Autodesk Inventor part; units mm, degrees
ref_plane "YZ Plane" through (0, 0, 0) normal (1, 0, 0) x (0, 1, 0)
ref_plane "XZ Plane" through (0, 0, 0) normal (0, 1, 0) x (-1, 0, 0)
ref_plane "XY Plane" through (0, 0, 0) normal (0, 0, 1) x (1, 0, 0)
sketch "Skizze1" plane through (0, 0, 0) normal (0, 0, 1) x (1, 0, 0)
  circle A0 centre (0.0001, -0.0022) radius 3.9802
  circle A1 centre (-8.37, 7.9978) radius 1.4
  circle A2 centre (8.3745, -8.0022) radius 1.4
  line L0 (-9.5383, 7.2264) -> (-3.2198, -2.3418)
  line L1 (-7.6522, 9.1998) -> (1.8915, 3.4999)
  line L2 (9.5428, -7.2307) -> (3.3215, 2.191)
  line L3 (-1.8517, -3.5253) -> (7.6567, -9.2041)
  point P0 (0, 0)
extrude "Extrusion1" add sketch "Skizze1" along normal blind 8
sketch "Skizze2" plane through (0, 0, 8) normal (0, 0, 1) x (1, 0, 0)
  arc A0 (-7.6522, 9.1998) -> (-9.5383, 7.2264) centre (-8.37, 7.9978) ccw
  line L0 (-9.5383, 7.2264) -> (-3.2198, -2.3418)
  arc A1 (-3.2198, -2.3418) -> (-1.8517, -3.5253) centre (0.0001, -0.0022) ccw
  line L1 (-1.8517, -3.5253) -> (7.6567, -9.2041)
  arc A2 (7.6567, -9.2041) -> (9.5428, -7.2307) centre (8.3745, -8.0022) ccw
  line L2 (9.5428, -7.2307) -> (3.3215, 2.191)
  arc A3 (3.3215, 2.191) -> (1.8915, 3.4999) centre (0.0001, -0.0022) ccw
  line L3 (1.8915, 3.4999) -> (-7.6522, 9.1998)
  arc A4 (-6.6267, 10.9169) -> (-11.2072, 6.1243) centre (-8.37, 7.9978) ccw
  line L4 (-11.2072, 6.1243) -> (-4.8666, -3.4774)
  arc A5 (-4.8666, -3.4774) -> (-2.8352, -5.2674) centre (0.0001, -0.0022) ccw
  line L5 (-2.8352, -5.2674) -> (6.6312, -10.9212)
  arc A6 (6.6312, -10.9212) -> (11.2118, -6.1287) centre (8.3745, -8.0022) ccw
  line L6 (11.2118, -6.1287) -> (4.9905, 3.2931)
  arc A7 (4.9905, 3.2931) -> (2.8837, 5.2369) centre (0.0001, -0.0022) ccw
  line L7 (2.8837, 5.2369) -> (-6.6267, 10.9169)
  point P0 (0, 0)
  dimension "d2" = 2
extrude "Extrusion2" add sketch "Skizze2" against normal up to surface (8 mm away)
sketch "Skizze3" plane through (0, 0, 8) normal (0, 0, 1) x (1, 0, 0)
  circle A0 centre (0.0001, -0.0022) radius 3.9802
  circle A1 centre (-8.37, 7.9978) radius 1.4
  circle A2 centre (8.3745, -8.0022) radius 1.4
  circle A3 centre (0.0001, -0.0022) radius 3.35
  point P0 (0, 0)
  dimension "d5" = 6.7
extrude "Extrusion3" cut sketch "Skizze3" against normal through all contours A1 | A2 | A3
sketch "Skizze4" plane through (0, 0, 8) normal (0, 0, 1) x (1, 0, 0)
  circle A0 centre (-8.37, 7.9978) radius 1.4
  circle A1 centre (8.3745, -8.0022) radius 1.4
  point P0 (0, 0)
hole "Bohrung1" at (-8.37, 7.9978, 8) at (8.3745, -8.0022, 8) direction (0, 0, -1) diameter 2.8 end through all counterbore diameter 8 counterbore depth 6
properties part number "IM_Lensholder"
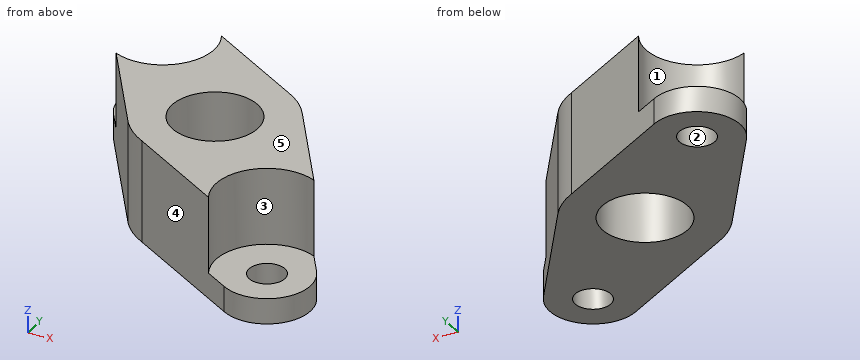
Read the model definition and answer for the solid it produces. Units are mm, in the model's axes. Face numbers are marked on the shaded views. A direction names the side the tool comes from. Coordinates: 2 decimals unless noted, no trailing zeros. Loops run counter-clockwise (first coordinate to the right, second up) from the corner with the lowest first, then second, coordinate; pieces in that order, holes last.
Q1. The part is cut by section B-B on x = 2. Write down the section's boundary in (y, z).
Q2. The mould has two halves that part along X. Classify the marked faces 3, 4 and 5: +X half, -X half, draft (parallel to the pull), parting line (faces both ways), or undercut.
Q3. Each of these flat-tipped pins is pushed along its axis until it touches: pin 1 Ø1 at (x, z) = (6, 2) entering from +Y; pin 2 Ø2 at (x, y) = (9, -9) entering from +Z; pin 3 Ø3 at (x, z) = (-6.5, 5) entering from -Y. Where does it stop, or does it pass through?
Q4. Which of the six approach directions +Z, -Z, +X, -X, +Y, -Y give full straight-line access (tool end or side, diameter ignored) to the marked faces 1 and 2?
Q5. The part is cut by section C-C on z = 1.5. Write down the section's boundary in (x, y).
Q6. The part is cut by section A-A on y = -2.5. Write down the section's boundary in (x, z).
Q7. The part is cut by section D-D on z = 5. Write down the section's boundary in (x, y).
Q8. Consider probe 1 along Z at (x, y) = (-6, 9.75); probe 2 along Y at (x, z) = (-8.37, 1.3); probe 3 along Y at (x, z) = (0, 7.75). Determine where each line is inside the solid, lowest interval first.
Results below:
1. outline: (-8.16, 0) - (-2.69, 0) - (-2.69, 8) - (-8.16, 8) - close; (2.69, 0) - (5.76, 0) - (5.76, 8) - (2.69, 8) - close
2. face 3: undercut
2. face 4: -X half
2. face 5: draft
3. pin 1: stops at y = 2.52
3. pin 2: stops at z = 2
3. pin 3: stops at y = -3.28
4. face 1: +Z
4. face 2: +Z, -Z
5. outline: (-11.21, 6.12) - (-4.87, -3.48) arc R5.98 ccw to (-2.84, -5.27) - (6.63, -10.92) arc R3.4 ccw to (11.21, -6.13) - (4.99, 3.29) arc R5.98 ccw to (2.88, 5.24) - (-6.63, 10.92) arc R3.4 ccw to start; hole circle Ø2.8 at (-8.37, 8); hole circle Ø6.7 at (0, 0); hole circle Ø2.8 at (8.37, -8)
6. outline: (-5.51, 0) - (-2.23, 0) - (-2.23, 8) - (-5.51, 8) - close; (2.23, 0) - (8.82, 0) - (8.82, 8) - (2.23, 8) - close
7. outline: (-10.05, 4.37) - (-4.87, -3.48) arc R5.98 ccw to (-2.84, -5.27) - (4.82, -9.84) arc R4 cw to (10.05, -4.37) - (4.99, 3.29) arc R5.98 ccw to (2.88, 5.24) - (-4.82, 9.84) arc R4 cw to start; hole circle Ø6.7 at (0, 0)
8. probe 1: z = 0 to 2
8. probe 2: y = 1.83 to 6.6, 9.4 to 11.4
8. probe 3: y = -6.96 to -3.35, 3.35 to 6.96
